Check sheet for the modelled part. Datum: model origin and axes. Units: mm. A direction names the side the tool comes from. Coordinates: 2 decimals unless noted, no trailing zeros. Loops run counter-clockwise (first coordinate to the right, second up) from the corner with the lowest first, then second, coordinate; pieces in that order, holes last. Notation, with made-up numbers: M 9,71 L 53,71 A29 ccw 53,107 Z; hole C 50,-14.5 d11. An arc over 180 degrees is marked long. Use CSV: the item, a comma, the result in double quotes. Start each with the question number.
(1) Section check C-C on y = 21.15. Record the cut outline in (x, z), and give its area (3 significant figures).
(2) Section check B-B on x = 43. Record the cut outline in (y, z).
(3) Section check D-D on z = -2.75. Record the cut outline in (x, y).
(4) Draft check along Z on faces 6 (the cylindrical face through (16.054, 24.754, 0.986)), 7 (the flat face through (3, 7, -13)), 8 (the cylindrical face through (0, 39, -10)). Enter one of: pulls with the +Z half, pulls with the -Z half, needs draft (parallel to the pull), parting line crosses it, or undercut.
(5) Scan lines: line 1 (X direction, y = 43.05, z = -10); line 2 (Y direction, x = 43, z = 2.5); line 3 (Y direction, x = 47, z = 1.4). Record each from-to range of solid material in increasing order.
(6) Set-up check for faces 1 (the flat face through (25, 18.7, 2)), 2 (the flat face through (-2, 45, -10)), 3 (the flat face through (55, 18, -8)), 4 (the flat face through (61, 41, -7.8)), 5 (the flat face through (-7, 41, -8)): record each of +Z, -Z, +X, -X, +Y, -Y from which the full face is reachable in a straight line by a thin tool's end or side.
(7) Go/stop test with flat-tipped pins: pin 1 Ø7 at (y, z) = (21.5, -3.5) entering from +X; pin 2 Ø8 at (x, z) = (60, -3) entering from -Y; pin 3 Ø6 at (x, z) = (-5, -10) entering from +Y. Record where each tip stops, or that it passes through.
(8) Section check A-A on y = 55. Record the cut outline in (x, z).
Autodesk Inventor part; units mm, degrees
ref_plane "YZ Plane" through (0, 0, 0) normal (1, 0, 0) x (0, 1, 0)
ref_plane "XZ Plane" through (0, 0, 0) normal (0, 1, 0) x (-1, 0, 0)
ref_plane "XY Plane" through (0, 0, 0) normal (0, 0, 1) x (1, 0, 0)
sketch "Sketch1" plane through (0, 0, 0) normal (0, 0, 1) x (1, 0, 0)
  line L0 (0, 0) -> (55, 0)
  line L1 (55, 0) -> (55, 65)
  line L2 (55, 65) -> (0, 65)
  line L3 (0, 65) -> (0, 0)
  dimension "d0" = 55
  dimension "d1" = 65
extrude "Extrusion1" add sketch "Sketch1" along normal blind 4
sketch "Sketch2" plane through (0, 0, 0) normal (0, 0, -1) x (-1, 0, 0)
  line L0 (0, 0) -> (-55, 0)
  line L1 (-55, 65) -> (0, 65)
  line L2 (-55, 0) -> (-55, 65)
  line L3 (0, 65) -> (0, 0)
  line L4 (0, 45) -> (-5, 45)
  line L5 (-5, 45) -> (-5, 0)
  line L6 (-55, 45) -> (-50, 45)
  line L7 (-50, 45) -> (-50, 0)
  dimension "d4" = 5
  dimension "d5" = 20
extrude "Extrusion2" add sketch "Sketch2" along normal blind 20 contours L0 L5 L4 L3 | L0 L2 L6 L7
sketch "Sketch3" plane through (0, 0, 4) normal (-1, 0, 0) x (0, 0, 1)
  line L0 (-4, 65) -> (-4, 45)
  line L1 (-4, 45) -> (-24, 45)
  line L2 (-4, 45) -> (-4, 41)
  line L3 (-4, 41) -> (-24, 41)
  line L4 (-24, 45) -> (-24, 0)
  point P0 (-4, 0)
  dimension "d8" = 4
extrude "Extrusion3" add sketch "Sketch3" along normal blind 10
sketch "Sketch4" plane through (55, 0, 4) normal (1, 0, 0) x (0, 0, -1)
  line L0 (24, 45) -> (24, 0)
  line L1 (4, 45) -> (24, 45)
  line L2 (4, 41) -> (24, 41)
  line L3 (4, 41) -> (4, 45)
  point P0 (4, 0)
extrude "Extrusion4" add sketch "Sketch4" along normal blind 10
sketch "Sketch5" plane through (0, 0, 0) normal (0, 0, -1) x (-1, 0, 0)
  line L0 (-5, 0) -> (-50, 0)
  line L1 (-5, 0) -> (-5, 45)
  circle A0 centre (-12, 5.65) radius 1.75
  circle A1 centre (-12, 36.65) radius 1.75
  circle A2 centre (-43, 5.65) radius 1.75
  circle A3 centre (-43, 36.65) radius 1.75
  point P0 (0, 0)
  dimension "d13" = 3.5
  dimension "d14" = 31
  dimension "d15" = 31
  dimension "d16" = 7
  dimension "d17" = 5.65
extrude "Extrusion5" cut sketch "Sketch5" against normal up to next
chamfer "Chamfer1" distance 14 angle 45 2 edges at (2.5, 0, -20) (52.5, 0, -20)
sketch "Sketch6" plane through (0, 0, 4) normal (0, 0, 1) x (1, 0, 0)
  line L0 (55, 0) -> (55, 65)
  line L1 (55, 65) -> (0, 65)
  line L2 (0, 65) -> (0, 0)
  circle A0 centre (8, 55) radius 2.25
  circle A1 centre (47, 55) radius 2.25
  dimension "d23" = 4.5
  dimension "d24" = 10
  dimension "d25" = 8
  dimension "d26" = 8
extrude "Extrusion6" cut sketch "Sketch6" against normal up to next
sketch "Sketch7" plane through (0, 41, -20) normal (0, -1, 0) x (1, 0, 0)
  line L0 (0, 20) -> (-10, 20)
  line L1 (-10, 0) -> (-10, 20)
  line L2 (55, 0) -> (55, 20)
  line L3 (55, 0) -> (65, 0)
  line L4 (65, 20) -> (65, 0)
  line L5 (55, 20) -> (65, 20)
  circle A0 centre (-5, 10) radius 2.25
  circle A1 centre (60, 10) radius 2.25
  dimension "d29" = 4.5
  dimension "d30" = 5
  dimension "d31" = 10
  dimension "d32" = 5
extrude "Extrusion7" cut sketch "Sketch7" against normal up to next contours A0 | A1
sketch "Sketch8" plane through (0, 41, 0) normal (0, 0, 1) x (1, 0, 0)
  line L0 (0, 4) -> (0, 0)
  line L1 (0, 4) -> (-10, 4)
  line L2 (-10, 0) -> (-10, 4)
  line L3 (0, 0) -> (-10, 0)
  line L4 (55, 0) -> (55, 4)
  line L5 (55, 0) -> (65, 0)
  line L6 (65, 4) -> (65, 0)
  line L7 (55, 4) -> (65, 4)
  point P0 (0, -41)
extrude "Extrusion8" add sketch "Sketch8" along normal up to surface (4 mm away)
sketch "Sketch9" plane through (0, 0, 4) normal (0, 0, 1) x (1, 0, 0)
  line L0 (55, 45) -> (65, 45)
  line L1 (55, 45) -> (55, 65)
  line L2 (0, 65) -> (0, 45)
  line L3 (-10, 45) -> (0, 45)
  line L4 (55, 65) -> (65, 45)
  line L5 (0, 65) -> (-10, 45)
extrude "Extrusion9" add sketch "Sketch9" against normal blind 4
sketch "Sketch10" plane through (0, 0, 0) normal (0, 0, -1) x (-1, 0, 0)
  circle A0 centre (-43, 5.65) radius 1.75
  circle A1 centre (-27.5, 21.15) radius 12
  point P0 (0, 0)
  dimension "d39" = 24
  dimension "d40" = 15.5
  dimension "d41" = 15.5
extrude "Extrusion10" cut sketch "Sketch10" against normal blind 2 contours A1
sketch "Sketch11" plane through (27.5, 21.15, 2) normal (0, 0, -1) x (-1, 0, 0)
  circle A0 centre (0, 0) radius 12
  circle A1 centre (0, 0) radius 3.25
  point P0 (27.5, -21.15)
  dimension "d44" = 6.5
extrude "Extrusion11" cut sketch "Sketch11" against normal up to next contours A1
chamfer "Chamfer2" distance 4 angle 45 2 edges at (0, 41, -8) (55, 41, -8)
sketch "Sketch12" plane through (-10, 41, -20) normal (0, -1, 0) x (1, 0, 0)
  arc A0 (6, 12.0156) -> (6, 7.9844) centre (5, 10) ccw
  line L0 (69, 12.0156) -> (69, 24)
  arc A1 (69, 7.9844) -> (69, 12.0156) centre (70, 10) ccw
  line L1 (69, 0) -> (69, 7.9844)
  line L2 (69, 0) -> (75, 0)
  line L3 (75, 0) -> (75, 24)
  line L4 (75, 24) -> (69, 24)
  circle A2 centre (5, 10) radius 5
  circle A3 centre (70, 10) radius 5
  point P0 (10, 20)
  dimension "d50" = 10
  dimension "d51" = 10
extrude "Extrusion12" cut sketch "Sketch12" along normal blind 7.5 contours A1 L1 A3 L0 | L0 A3 L1 A1 | A2
properties part number "ZMotorMount" material "ABS Plastic"
Outcome:
1,outline,"M 0,-20 L 5,-20 L 5,0 L 15.5,0 L 15.5,2 L 24.25,2 L 24.25,4 L 0,4 Z; M 30.75,2 L 39.5,2 L 39.5,0 L 50,0 L 50,-20 L 55,-20 L 55,4 L 30.75,4 Z"
1,area,"359 mm²"
2,outline,"M 0,0 L 3.9,0 L 3.9,4 L 0,4 Z; M 7.4,0 L 34.9,0 L 34.9,4 L 7.4,4 Z; M 38.4,0 L 65,0 L 65,4 L 38.4,4 Z"
3,outline,"M -10,41 L -4,41 L 0,37 L 0,0 L 5,0 L 5,45 L -10,45 Z; M 50,0 L 55,0 L 55,37 L 59,41 L 65,41 L 65,45 L 50,45 Z"
4,face 6,"needs draft"
4,face 7,"pulls with the -Z half"
4,face 8,"undercut"
5,line 1,"x = -10 to -7.25, -2.75 to 5, 50 to 57.75, 62.25 to 65"
5,line 2,"y = 0 to 3.9, 7.4 to 34.9, 38.4 to 65"
5,line 3,"y = 0 to 52.75, 57.25 to 65"
6,face 1,"-Z"
6,face 2,"-Z, +X, -X, +Y"
6,face 3,"+Z, -Z, +X, -Y"
6,face 4,"+X, -Y"
6,face 5,"-X, -Y"
7,pin 1,"stops at x = 55"
7,pin 2,"stops at y = 38"
7,pin 3,"stops at y = 45"
8,outline,"M -5,0 L 5.75,0 L 5.75,4 L -5,4 Z; M 10.25,0 L 44.75,0 L 44.75,4 L 10.25,4 Z; M 49.25,0 L 60,0 L 60,4 L 49.25,4 Z"
